from build123d import *

# Parameters (mm, degrees)
F0_W     = 114.3
F0_H     = 76.2
F1_DEPTH = 3.175
F2_W     = 114.3
F2_H     = 76.2
F2_W_2   = 107.95
F2_H_2   = 69.85
F3_DEPTH = 25.4
F5_W     = 7.62
F5_H     = 7.62
F6_DEPTH = 11.43
F7_SIZE  = 6.35


with BuildPart() as f1:
    # F0 (on Top) → F1 (new body)
    with BuildSketch(Plane.XY):
        Rectangle(F0_W, F0_H)
    extrude(amount=F1_DEPTH)

    # F2 (on face) → F3 (join)
    with BuildSketch(Plane.XY.offset(3.175)):
        Rectangle(F2_W, F2_H)
        Rectangle(F2_W_2, F2_H_2, mode=Mode.SUBTRACT)
    extrude(amount=F3_DEPTH)

    # F5 (on offset) → F6 (join)
    with BuildSketch(Plane.XY.offset(23.495)):
        with Locations((-50.967861, 28.804621)):
            Rectangle(F5_W, F5_H)
    extrude(amount=-F6_DEPTH)

    # F7
    f7_edges = [f1.edges().sort_by_distance(p)[0] for p in [
        (-47.157861, 28.804621, 12.065),
    ]]
    chamfer(f7_edges, length=F7_SIZE)


solid = f1.part
For this review, take the finished solid that the model builds, in its own axes (mm). A direction names the side the tool comes from. Coordinates: 2 decimals unless noted, no trailing zeros. Write each loop counter-clockwise with the first axis right and the second up, starting at its lowest first coordinate (ties: lowest second). Pieces come first, ordered by that corner, then holes. Notation, with made-up numbers: (12, 88) -> (48, 88) arc R20 cw to (48, 110) -> close; hole circle Ø4 at (-30.5, -2). An arc over 180 degrees is marked (long way). Write each question's results on one line, items separated by ' | '. Start each with the question number.
1) Consider section D-D (z = 5.5). Write out the cut boundary in (x, y) (3 decimals), plus the area to 3 significant figures.
2) Wall thickness on L1, parallel to X at y = 29, z = 10.5 (3 decimals); L2, parallel to Y at x = 26.5, z = 21.5 (3 decimals); L3, parallel to Z at x = -6, y = 6 (3 decimals): over which ranges is each line inside the solid? List them lowest first. Write a range as [from, to].
3) Consider section C-C (y = 30). Write out the cut boundary in (x, z) (3 decimals), plus the area to 3 significant figures.
4) Consider section B-B (x = 0). Write out the cut boundary in (y, z) (3 decimals), plus the area to 3 significant figures.
5) For faces 5 (the face through (-5, -37, 28.575)), 6 (the face through (-51, 32.615, 19)), list the 3-axis set-ups (+Z, -Z, +X, -X, +Y, -Y) from which the entire face can be reached by the end or side of a thin tool; tool diameter is ignored.
6) Insertion check: pin 1 (8 mm diameter, centred on x = -30.5, y = 24, fed in from +Z) (3 decimals). The pin has a flat end and moves straight along its axis. Give the tip position at first contact, or say it passes through.
7) The part is to be moulded in two halves that separate along X. For faces 1 (the face through (-50.377, 28.751, 15.196)), 2 (the face through (-1, -34.925, 16)), 3 (the face through (-1, 38.1, 14)), 4 (the face through (-57.15, -1, 14)), say which applies: +X half, -X half, draft (parallel to the pull), parting line (faces both ways), or undercut.
8) Consider section A-A (z = 21.25). Write out the cut boundary in (x, y) (3 decimals).
Geometry says:
1) outline: (-57.15, -38.1) -> (57.15, -38.1) -> (57.15, 38.1) -> (-57.15, 38.1) -> close; hole (-53.975, -34.925) -> (53.975, -34.925) -> (53.975, 34.925) -> (-53.975, 34.925) -> close | area: 1,170 mm^2
2) L1: [-57.15, -53.975], [53.975, 57.15] | L2: [-38.1, -34.925], [34.925, 38.1] | L3: [0, 3.175]
3) outline: (-57.15, 0) -> (57.15, 0) -> (57.15, 28.575) -> (53.975, 28.575) -> (53.975, 3.175) -> (-53.975, 3.175) -> (-53.975, 12.065) -> (-53.508, 12.065) -> (-47.158, 18.415) -> (-47.158, 23.495) -> (-53.975, 23.495) -> (-53.975, 28.575) -> (-57.15, 28.575) -> close | area: 582 mm^2
4) outline: (-38.1, 0) -> (38.1, 0) -> (38.1, 28.575) -> (34.925, 28.575) -> (34.925, 3.175) -> (-34.925, 3.175) -> (-34.925, 28.575) -> (-38.1, 28.575) -> close | area: 403 mm^2
5) face 5: +Z, +X, -X, +Y, -Y | face 6: +Z
6) pin 1: z = 3.175
7) face 1: undercut | face 2: undercut | face 3: draft | face 4: -X half
8) outline: (-57.15, -38.1) -> (57.15, -38.1) -> (57.15, 38.1) -> (-57.15, 38.1) -> close; hole (-53.975, -34.925) -> (53.975, -34.925) -> (53.975, 34.925) -> (-53.975, 34.925) -> (-53.975, 32.615) -> (-47.158, 32.615) -> (-47.158, 24.995) -> (-53.975, 24.995) -> close
